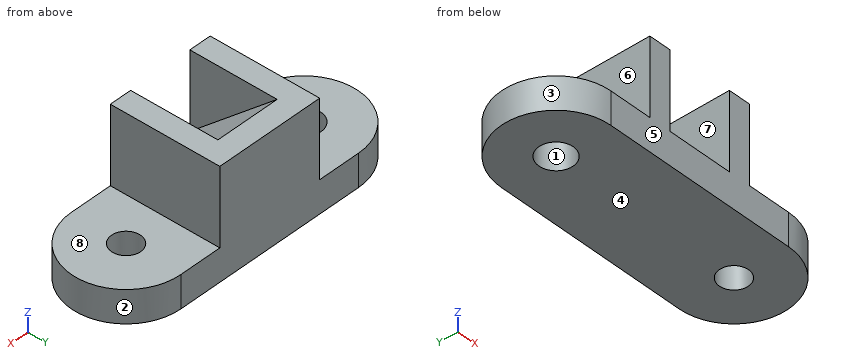
Autodesk Fusion 360 part; units mm, degrees
sketch "Sketch1" plane through (0, 0, 0) normal (0, 0, 1) x (1, 0, 0)
  line L0 (0, 0) -> (114, 0)
  line L1 (114, 0) -> (114, 64)
  line L2 (114, 64) -> (0, 64)
  line L3 (0, 64) -> (0, 0)
  dimension "d1" = 114
  dimension "d2" = 64
extrude "Extrude1" add sketch "Sketch1" along normal blind 19
sketch "Sketch2" plane through (0, 0, 19) normal (0, 0, 1) x (-1, 0, 0)
  line L0 (0, -64) -> (0, 0)
  line L1 (0, 0) -> (-114, 0)
  line L2 (-114, 0) -> (-114, -64)
  line L3 (-114, -64) -> (0, -64)
  line L4 (0, 0) -> (-25, 0)
  line L5 (-25, 0) -> (-89, 0)
  line L6 (-89, 0) -> (-89, -64)
  line L7 (-89, -64) -> (-25, -64)
  line L8 (-25, -64) -> (-25, 0)
  dimension "d5" = 25
  dimension "d6" = 64
extrude "Extrude2" add sketch "Sketch2" along normal blind 45 contours L1 L3 L5 L6 L7 L8
sketch "Sketch4" plane through (0, 0, 64) normal (0, 0, 1) x (-1, 0, 0)
  line L0 (-25, -64) -> (-25, 0)
  line L1 (-25, 0) -> (-89, 0)
  line L2 (-89, 0) -> (-89, -64)
  line L3 (-89, -64) -> (-25, -64)
  line L4 (-25, 0) -> (-38, 0)
  line L5 (-38, 0) -> (-38, -51)
  line L6 (-38, -51) -> (-76, -51)
  line L7 (-76, -51) -> (-76, 0)
  line L8 (-38, 0) -> (-76, 0)
  dimension "d12" = 13
  dimension "d13" = 51
  dimension "d14" = 38
extrude "Extrude3" cut sketch "Sketch4" against normal blind 45 contours L1 L5 L6 L7 L8
sketch "Sketch5" plane through (38, 0, 0) normal (1, 0, 0) x (0, 1, 0)
  line L0 (51, 64) -> (0, 64)
  line L1 (0, 64) -> (0, 19)
  line L2 (0, 19) -> (51, 19)
  line L3 (51, 19) -> (51, 64)
  line L4 (51, 64) -> (0, 19)
  line L5 (51, 19) -> (0, 19)
  line L6 (51, 19) -> (51, 64)
extrude "Extrude4" add sketch "Sketch5" along normal blind 38 contours L2 L3 L4 L5 L6
sketch "Sketch6" plane through (0, 0, 19) normal (0, 0, 1) x (-1, 0, 0)
  line L0 (-89, -64) -> (-89, 0)
  line L1 (-89, 0) -> (-114, 0)
  line L2 (-114, 0) -> (-114, -64)
  line L3 (-114, -64) -> (-89, -64)
  circle A0 centre (-114, -32) radius 32
  line L4 (-114, -64) -> (-114, 0)
  dimension "d31" = 64
extrude "Extrude5" add sketch "Sketch6" against normal blind 19 contours L2 A0 L4
hole "Hole1" at (114, 32, 19) direction (0, 0, -1) diameter 17 depth 22 tip angle 118
sketch "Sketch7" plane through (0, 0, 19) normal (0, 0, 1) x (-1, 0, 0)
  line L0 (-25, 0) -> (-25, -64)
  line L1 (-25, -64) -> (0, -64)
  line L2 (0, -64) -> (0, 0)
  line L3 (0, 0) -> (-25, 0)
  circle A0 centre (0, -32) radius 32
  line L4 (0, -64) -> (0, 0)
  dimension "d25" = 64
extrude "Extrude6" add sketch "Sketch7" against normal blind 19 contours L2 A0 L4
hole "Hole2" at (0, 32, 19) direction (0, 0, -1) diameter 20 depth 22 tip angle 118
CAD build for the part. Positions are in the model's coordinates, mm. Face numbers are marked on the shaded views. A direction names the side the tool comes from. Give positions to 0.01 mm unless a question says otherwise; leave off trailing zeros. Order: outer loops, then holes, each group sorted by start corner. A loop starts at its lowest first (then second) coordinate and runs counter-clockwise, first axis right, second up. Notation, with made-up numbers: (51, 25.25) - (87, 25.25) arc R21 cw to (87, 45.25) - close; hole circle Ø2 at (37.25, 70). An arc over 180 degrees is marked (long way). Write each question's results on one line, items separated by ' | '.
1. Probe L1, parallel to X at y = 32, z = 14.5; L2, parallel to Y at x = 0, z = 4; L3, parallel to Y at x = 114, z = 15.25. List the from-to ranges inside material, lowest first. Write a range as from..to.
Calculated:
L1: x = -32..-10, 10..105.5, 122.5..146 | L2: y = 0..22, 42..64 | L3: y = 0..23.5, 40.5..64
2. Saw through at C-C on x = 44. List the corners of the cut face in (y, z), and give its area (3 significant figures).
Calculated:
outline: (0, 0) - (64, 0) - (64, 64) - (51, 64) - (0, 19) - close | area: 2,950 mm2
3. Pull direction X, two halves, no side cores. Call the marked faces 1, 2, 3 and 4: released by +X, released by -X, zero draft, split by the parting line, or undercut.
Calculated:
face 1: undercut | face 2: released by +X | face 3: released by -X | face 4: zero draft
4. Saw through at D-D on x = 119.5. List the corners of the cut face in (y, z), and give its area (3 significant figures).
Calculated:
outline: (0.48, 0) - (25.52, 0) - (25.52, 19) - (0.48, 19) - close; (38.48, 0) - (63.52, 0) - (63.52, 19) - (38.48, 19) - close | area: 952 mm2
5. 3-axis set-ups, long thin cutter, end or side, ignore diameter. For the marked faces 5, 6, 7 and 8: which of +Z, -Z, +X, -X, +Y, -Y reach the whole face in a straight line?
Calculated:
face 5: +Z, -Z, +X, -X, -Y | face 6: +Z, -X, +Y, -Y | face 7: +Z, -Y | face 8: +Z, +X, +Y, -Y
6. Saw through at B-B on y = 36. List the corners of the cut face in (x, z), and give its area (3 significant figures).
Calculated:
outline: (-31.75, 0) - (-9.17, 0) - (-9.17, 19) - (-31.75, 19) - close; (9.17, 0) - (106.5, 0) - (106.5, 19) - (89, 19) - (89, 64) - (76, 64) - (76, 50.76) - (38, 50.76) - (38, 64) - (25, 64) - (25, 19) - (9.17, 19) - close; (121.5, 0) - (145.75, 0) - (145.75, 19) - (121.5, 19) - close | area: 5,120 mm2
7. Pin check, flat tips, straight feed: pin 1 (1 mm diameter, centred on x = 111, y = 49, fed in from +Z); pin 2 (8 mm diameter, centred on x = 19, y = 7, fed in from -Z); pin 3 (18 mm diameter, centred on x = 0, y = 32, fed in from -Z); pin 4 (12 mm diameter, centred on y = 44.5, z = 53.5, fed in from -X). Stop position of each tip, or through.
Calculated:
pin 1: stops at z = 19 | pin 2: stops at z = 0 | pin 3: passes through | pin 4: stops at x = 25
8. Saw through at A-A on z = 35.5. List the corners of the cut face in (x, y).
Calculated:
outline: (25, 0) - (38, 0) - (38, 18.7) - (76, 18.7) - (76, 0) - (89, 0) - (89, 64) - (25, 64) - close
